Check sheet for the modelled part. Datum: model origin and axes. Units: mm. Face numbers are marked on the shaded views. Give positions to 0.01 mm unless a question says otherwise; leave off trailing zeros. Write each loop counter-clockwise with the first axis right and the second up, starting at its lowest first coordinate (ties: lowest second). Pieces come first, ordered by that corner, then holes. Notation, with made-up numbers: (28, 46) -> (55, 46) arc R33 ccw to (55, 82) -> close; hole circle Ø9 at (69.5, -26). An arc over 180 degrees is marked (long way). Return JSON: item names as keys, results as strings.
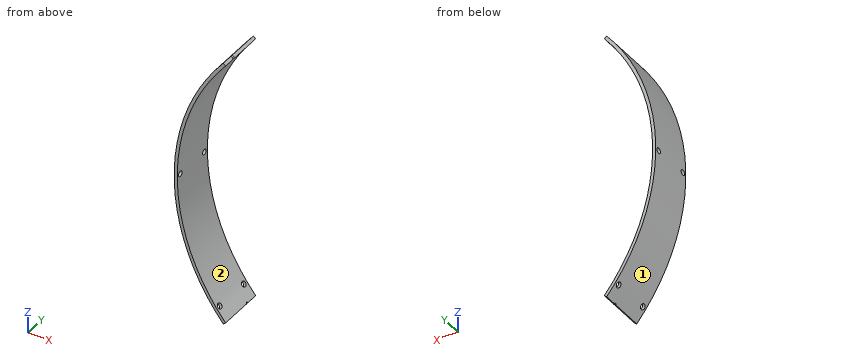
from build123d import *

# Parameters (mm, degrees)
SKETCH1_W                       = 1.5
SKETCH1_H                       = 22.7
REVOLVE1_ANGLE                  = 80
SKETCH2_R                       = 1.3125
CUT_EXTRUDE1_DEPTH              = 122.192879456
CIRPATTERN1_COUNT               = 2
CIRPATTERN1_ANGLE               = 36
CIRPATTERN1_THE_OTHER_WAY_COUNT = 2
CIRPATTERN1_THE_OTHER_WAY_ANGLE = 36
CUT_EXTRUDE2_DEPTH              = 133.380069744
CUT_EXTRUDE2_DEPTH_BACK         = 133.380069744
SKETCH3_R                       = 0.5
CUT_EXTRUDE3_DEPTH              = 133.380069744
CUT_EXTRUDE3_DEPTH_BACK         = 133.380069744
SKETCH4_R                       = 0.5


with BuildPart() as part:
    # Sketch1 → Revolve1 (revolve, symmetric)
    with BuildSketch(Plane.XY) as revolve1_sk:
        with Locations((-100.75, 0)):
            Rectangle(SKETCH1_W, SKETCH1_H)
    revolve(axis=Axis((0, -1000, 0), (0, 1, 0)), revolution_arc=REVOLVE1_ANGLE / 2)
    revolve(revolve1_sk.sketch, axis=Axis((0, -1000, 0), (0, -1, 0)), revolution_arc=REVOLVE1_ANGLE / 2)

    # Sketch2 → Cut-Extrude1 (cut, through all)
    with BuildSketch(Plane(origin=(0, 0, 0), x_dir=(0, 0, -1), z_dir=(1, 0, 0))):
        with Locations((0, -9.1)):
            Circle(SKETCH2_R)
        with Locations((0, 9.1)):
            Circle(SKETCH2_R)
    cut_extrude1 = extrude(amount=-CUT_EXTRUDE1_DEPTH, mode=Mode.SUBTRACT)

    # CirPattern1: Cut-Extrude1 ×2 about axis
    cirpattern1_axis = Axis((0, -1000, 0), (0, 1, 0))
    for i in range(1, CIRPATTERN1_COUNT):
        add(cut_extrude1.rotate(cirpattern1_axis, i * CIRPATTERN1_ANGLE / (CIRPATTERN1_COUNT - 1)), mode=Mode.SUBTRACT)

    # CirPattern1 the other way: Cut-Extrude1 ×2 about axis
    cirpattern1_the_other_way_axis = Axis((0, -1000, 0), (0, -1, 0))
    for i in range(1, CIRPATTERN1_THE_OTHER_WAY_COUNT):
        add(cut_extrude1.rotate(cirpattern1_the_other_way_axis, i * CIRPATTERN1_THE_OTHER_WAY_ANGLE / (CIRPATTERN1_THE_OTHER_WAY_COUNT - 1)), mode=Mode.SUBTRACT)

    # Sketch3 → Cut-Extrude2 (cut, two sides: drawn at the far end of the back side and taken through both)
    with BuildSketch(Plane(origin=(-76.604444312, 0, 64.278760969), x_dir=(-0.6427876096865407, 0, -0.7660444431189769), z_dir=(0.7660444431189769, -1.1789167470557806e-15, -0.6427876096865407)).offset(-CUT_EXTRUDE2_DEPTH_BACK)):
        with Locations((0, -5)):
            Circle(SKETCH3_R)
    extrude(amount=CUT_EXTRUDE2_DEPTH + CUT_EXTRUDE2_DEPTH_BACK, mode=Mode.SUBTRACT)

    # Sketch4 → Cut-Extrude3 (cut, two sides: drawn at the far end of the back side and taken through both)
    with BuildSketch(Plane(origin=(-76.604444312, 0, -64.278760969), x_dir=(-0.6427876096865405, 0, 0.7660444431189771), z_dir=(-0.7660444431189772, 0, -0.6427876096865405)).offset(-CUT_EXTRUDE3_DEPTH_BACK)):
        with Locations((-1e-09, 5)):
            Circle(SKETCH4_R)
    extrude(amount=CUT_EXTRUDE3_DEPTH + CUT_EXTRUDE3_DEPTH_BACK, mode=Mode.SUBTRACT)


solid = part.part
(1) Cross-section at B-B on x = -94.75. Enter the section's corners in (y, z).
Reply:
{"outline": "(-11.35, -36.4) -> (11.35, -36.4) -> (11.35, -31.98) -> (-11.35, -31.98) -> close; (-11.35, 31.98) -> (11.35, 31.98) -> (11.35, 36.4) -> (-11.35, 36.4) -> close"}
(2) Thickness scan on L1, parallel to Z at x = -79.25, y = 2.75; L2, parallel to Z at x = -81.75, y = -4.5; L3, parallel to X at y = 2.5, z = 33. Record the ranges inside material, lowest first.
Reply:
{"L1": "-63.42 to -60.99, 60.99 to 63.42", "L2": "-60.16 to -57.59, 57.59 to 60.16", "L3": "-95.99 to -94.4"}
(3) Cross-section at A-A on z = 0. Enter the section's corners in (x, y).
Reply:
{"outline": "(-101.5, -11.35) -> (-100, -11.35) -> (-100, -10.41) -> (-101.5, -10.41) -> close; (-101.5, -7.79) -> (-100, -7.79) -> (-100, 7.79) -> (-101.5, 7.79) -> close; (-101.5, 10.41) -> (-100, 10.41) -> (-100, 11.35) -> (-101.5, 11.35) -> close"}
(4) Cross-section at D-D on x = -89.25. Enter the section's corners in (y, z), then the cut area to 3 significant figures.
Reply:
{"outline": "(-11.35, -48.34) -> (11.35, -48.34) -> (11.35, -45.1) -> (-11.35, -45.1) -> close; (-11.35, 45.1) -> (11.35, 45.1) -> (11.35, 48.34) -> (-11.35, 48.34) -> close", "area": "147 mm^2"}
(5) Release check for a two-part mould opening along Z. For the marked faces 1 and 2 record: pulls with the +Z half, pulls with the -Z half, needs draft (parallel to the pull), parting line crosses it, or undercut.
Reply:
{"face 1": "parting line crosses it", "face 2": "undercut"}
(6) Cross-section at C-C on y = 9.1. Enter the section's corners in (x, z), then the cut area to 3 significant figures.
Reply:
{"outline": "(-101.49, -1.31) arc R101.5 ccw to (-82.88, -58.59) -> (-81.67, -57.71) arc R100 cw to (-99.99, -1.31) -> close; (-101.49, 1.31) -> (-99.99, 1.31) arc R100 cw to (-81.67, 57.71) -> (-82.88, 58.59) arc R101.5 ccw to start; (-81.34, -60.72) arc R101.5 ccw to (-77.75, -65.24) -> (-76.6, -64.28) arc R100 cw to (-80.12, -59.84) -> close; (-81.34, 60.72) -> (-80.12, 59.84) arc R100 cw to (-76.6, 64.28) -> (-77.75, 65.24) arc R101.5 ccw to start", "area": "199 mm^2"}
(7) Depth check by flat-ended pin: pin 1 Ø12 at (x, y) = (-79, 7.5) entering from +Z; pin 2 Ø3 at (y, z) = (9.1, 0) entering from +X; pin 3 Ø8 at (x, y) = (-82, 4) entering from -Z; pin 4 Ø1.6 at (y, z) = (-9.1, 0) entering from -X. Enter the tip coordinate at first touch or a pass-through.
Reply:
{"pin 1": "z = 65.24", "pin 2": "x = -99.99", "pin 3": "z = -64.95", "pin 4": "through"}
